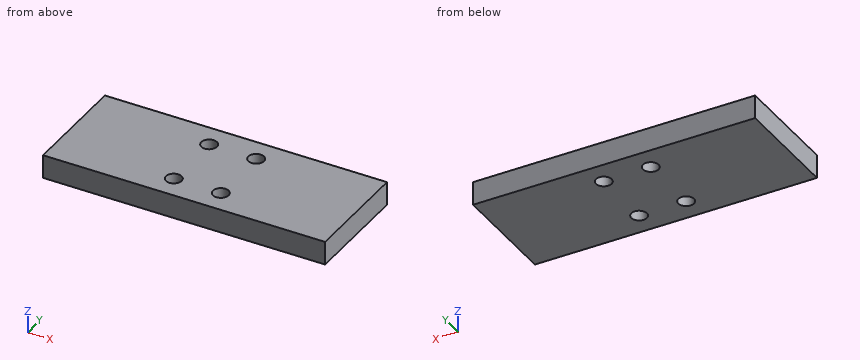
```python
from build123d import *

# Parameters (mm, degrees)
SKETCH_1_W      = 180
SKETCH_1_H      = 70
SKETCH_1_R      = 5
EXTRUDE_1_DEPTH = 7.5


with BuildPart() as part:
    # 草图1 → 凸台-拉伸1 (new, symmetric)
    with BuildSketch(Plane.XY):
        Rectangle(SKETCH_1_W, SKETCH_1_H)
        with Locations((-15, 20)):
            Circle(SKETCH_1_R, mode=Mode.SUBTRACT)
        with Locations(Location((15, 20, 0), (0, 0, 180))):
            Circle(SKETCH_1_R, mode=Mode.SUBTRACT)
        with Locations((15, -20)):
            Circle(SKETCH_1_R, mode=Mode.SUBTRACT)
        with Locations(Location((-15, -20, 0), (0, 0, 180))):
            Circle(SKETCH_1_R, mode=Mode.SUBTRACT)
    extrude(amount=EXTRUDE_1_DEPTH, both=True)


solid = part.part
```
Design review of the part built by this model. Coordinates are the model's own, in mm. Give positions to 0.01 mm unless a question says otherwise; leave off trailing zeros. Loops run counter-clockwise (first coordinate to the right, second up) from the corner with the lowest first, then second, coordinate; pieces in that order, holes last. Notation, with made-up numbers: (16, 0.5) -> (34, 0.5) arc R9 cw to (34, 11.5) -> close; hole circle Ø5 at (-27, 87.25). An arc over 180 degrees is marked (long way). One line per item, written item: value.
Q1. We need section B-B on y = 20. Give the boundary of the cut face in (x, z), and give its area (3 significant figures).
Numbers:
outline: (-90, -7.5) -> (-20, -7.5) -> (-20, 7.5) -> (-90, 7.5) -> close; (-10, -7.5) -> (10, -7.5) -> (10, 7.5) -> (-10, 7.5) -> close; (20, -7.5) -> (90, -7.5) -> (90, 7.5) -> (20, 7.5) -> close
area: 2,400 mm^2
Q2. We need section A-A on x = 15. Give the boundary of the cut face in (y, z).
Numbers:
outline: (-35, -7.5) -> (-25, -7.5) -> (-25, 7.5) -> (-35, 7.5) -> close; (-15, -7.5) -> (15, -7.5) -> (15, 7.5) -> (-15, 7.5) -> close; (25, -7.5) -> (35, -7.5) -> (35, 7.5) -> (25, 7.5) -> close
Q3. For L1, parallel to Y at x = -15, z = -2.25; L2, parallel to X at y = 21, z = 5, list the stretches that pass through material, from the lowest coordinate up.
Numbers:
L1: y = -35 to -25, -15 to 15, 25 to 35
L2: x = -90 to -19.9, -10.1 to 10.1, 19.9 to 90
Q4. We need section C-C on z = 0. Give the boundary of the cut face in (x, y).
Numbers:
outline: (-90, -35) -> (90, -35) -> (90, 35) -> (-90, 35) -> close; hole circle Ø10 at (-15, -20); hole circle Ø10 at (-15, 20); hole circle Ø10 at (15, -20); hole circle Ø10 at (15, 20)
